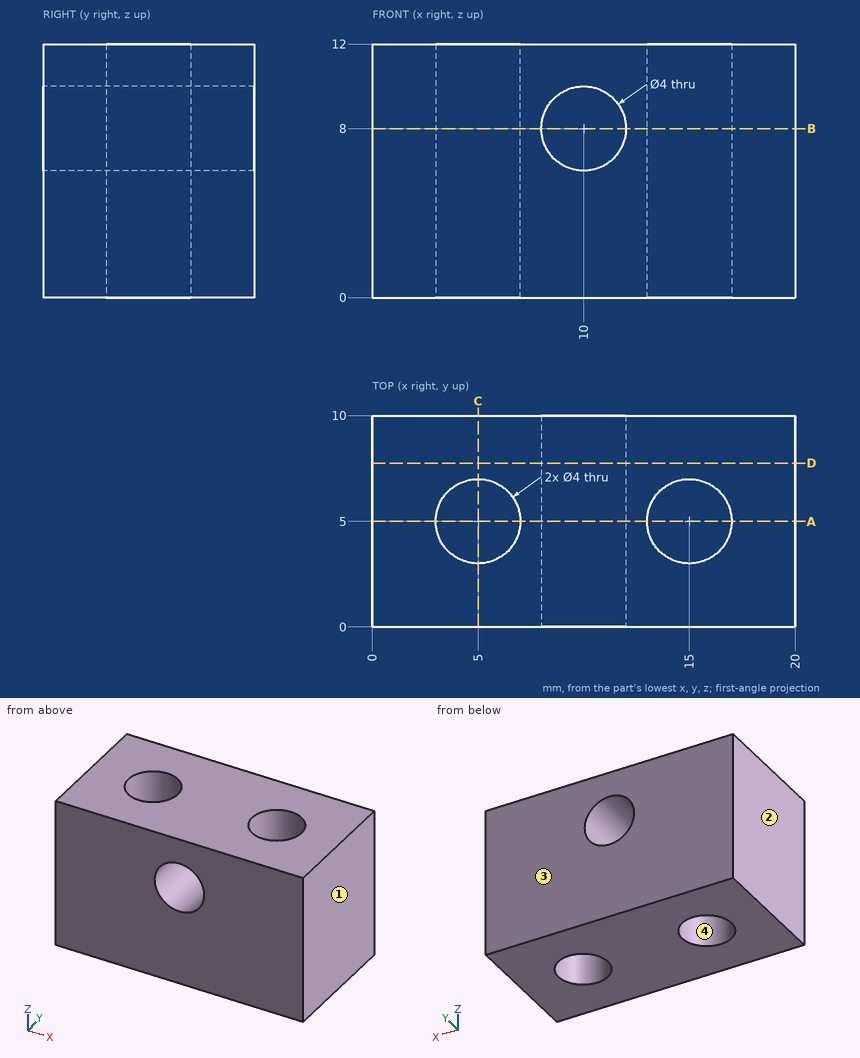
Answer from the drawing. Dimensions are ordinates in mm from the lowest x, y and z of the part. Give positions to 0.01 mm unless a question says otherwise; leave off trailing zeros. Loops run counter-clockwise (first coordinate to the right, second up) from the corner with the lowest first, then second, coordinate; pieces in that order, holes last.
Item 1: The part is cut by section C-C (x = 5). Write down the section's boundary in (y, z), and give its area (3 significant figures).
Item 2: Find the intervals of material crossed by line 1 along X through (y, z) = (2.75, 8); line 2 along Y through (x, z) = (15, 5.75); line 3 along X through (y, z) = (5.75, 10.75), in increasing order.
Item 3: The part is cut by section D-D (y = 7.75). Write down the section's boundary in (x, z), and give its area (3 significant figures).
Item 4: The mould has two halves that part along X. Classify the marked faces 1, 2, 3 and 4: released by +X, released by -X, zero draft, split by the parting line, or undercut.
Item 5: The part is cut by section A-A (y = 5). Write down the section's boundary in (x, z), and give its area (3 significant figures).
Item 6: The part is cut by section B-B (z = 8). Write down the section's boundary in (x, y), and give its area (3 significant figures).
Taken from the geometry:
1. outline: (0, 0) - (3, 0) - (3, 12) - (0, 12) - close; (7, 0) - (10, 0) - (10, 12) - (7, 12) - close
1. area: 72.0 mm2
2. line 1: x = 0 to 8, 12 to 20
2. line 2: y = 0 to 3, 7 to 10
2. line 3: x = 0 to 3.15, 6.85 to 13.15, 16.85 to 20
3. outline: (0, 0) - (20, 0) - (20, 12) - (0, 12) - close; hole circle Ø4 at (10, 8)
3. area: 227 mm2
4. face 1: released by +X
4. face 2: released by -X
4. face 3: zero draft
4. face 4: undercut
5. outline: (0, 0) - (3, 0) - (3, 12) - (0, 12) - close; (7, 0) - (13, 0) - (13, 12) - (7, 12) - close; (17, 0) - (20, 0) - (20, 12) - (17, 12) - close; hole circle Ø4 at (10, 8)
5. area: 131 mm2
6. outline: (0, 0) - (8, 0) - (8, 10) - (0, 10) - close; (12, 0) - (20, 0) - (20, 10) - (12, 10) - close; hole circle Ø4 at (5, 5); hole circle Ø4 at (15, 5)
6. area: 135 mm2
